Can you work these out from the model? Positions are in its coordinate system, mm. Face numbers are marked on the shaded views. A direction names the side the tool comes from. Round coordinates to 2 decimals unless told otherwise and drop trailing zeros. Order: outer loops, then holes, each group sorted by start corner. A loop starts at its lowest first (then second) coordinate and runs counter-clockwise, first axis right, second up. Notation, with made-up numbers: M -32,3 L 18,3 A16 cw 18,15 Z; hole C 57.25,60 d3. An arc over 180 degrees is marked long. Answer as a JSON object with one key per item and string values. Group by question number.
from build123d import *

# Parameters (mm, degrees)
SKETCH1_W           = 42.3
SKETCH1_H           = 42.3
BOSS_EXTRUDE1_DEPTH = 46.9
SKETCH2_W           = 39
SKETCH2_H           = 39
BOSS_EXTRUDE2_DEPTH = 4.85
SKETCH3_R           = 17.6
BOSS_EXTRUDE3_DEPTH = 15.88
SKETCH4_R           = 17.6
BOSS_EXTRUDE4_DEPTH = 6.5
SKETCH5_R           = 10.75
BOSS_EXTRUDE5_DEPTH = 2.15
SKETCH6_R           = 4
BOSS_EXTRUDE6_DEPTH = 17.5
CUT_EXTRUDE1_DEPTH  = 13.5
CHAMFER1_SIZE       = 3
CHAMFER2_SIZE       = 1
FILLET1_R           = 1


with BuildPart() as part:
    # Sketch1 → Boss-Extrude1 (new body)
    with BuildSketch(Plane.XY):
        Rectangle(SKETCH1_W, SKETCH1_H)
    extrude(amount=BOSS_EXTRUDE1_DEPTH)

    # Sketch2 → Boss-Extrude2 (add)
    with BuildSketch(Plane.XY.offset(46.9)):
        Rectangle(SKETCH2_W, SKETCH2_H)
    extrude(amount=BOSS_EXTRUDE2_DEPTH)

    # Sketch3 → Boss-Extrude3 (add)
    with BuildSketch(Plane.XY.offset(51.75)):
        Circle(SKETCH3_R)
    extrude(amount=BOSS_EXTRUDE3_DEPTH)

    # Sketch4 → Boss-Extrude4 (add)
    with BuildSketch(Plane.XY.offset(67.63)):
        Circle(SKETCH4_R)
    extrude(amount=BOSS_EXTRUDE4_DEPTH)

    # Sketch5 → Boss-Extrude5 (add)
    with BuildSketch(Plane.XY.offset(74.13)):
        with Locations(Location((0, 0, 0), (0, 0, 180))):
            Circle(SKETCH5_R)
    extrude(amount=BOSS_EXTRUDE5_DEPTH)

    # Sketch6 → Boss-Extrude6 (add)
    with BuildSketch(Plane.XY.offset(76.28)):
        Circle(SKETCH6_R)
    extrude(amount=BOSS_EXTRUDE6_DEPTH)

    # Sketch7 → Cut-Extrude1 (cut)
    with BuildSketch(Plane.XY.offset(93.78)):
        Polygon((-80.453133814, 3), (-2.645751311, 3), (2.645751311, 3), (80.453133814, 3), (80.453133814, 158.614765005), (-80.453133814, 158.614765005), align=None)
    extrude(amount=-CUT_EXTRUDE1_DEPTH, mode=Mode.SUBTRACT)

    # Chamfer1
    chamfer1_edges = [part.edges().sort_by_distance(p)[0] for p in [
        (19.5, -19.5, 49.325),
        (19.5, 19.5, 49.325),
        (-19.5, 19.5, 49.325),
        (-19.5, -19.5, 49.325),
        (-21.15, -21.15, 23.45),
        (21.15, -21.15, 23.45),
        (21.15, 21.15, 23.45),
        (-21.15, 21.15, 23.45),
    ]]
    chamfer(chamfer1_edges, length=CHAMFER1_SIZE)

    # Chamfer2
    chamfer2_edges = [part.edges().sort_by_distance(p)[0] for p in [
        (-19.5, 0, 51.75),
        (0, 19.5, 51.75),
        (19.5, 0, 51.75),
        (0, -19.5, 51.75),
        (18, 18, 51.75),
        (18, -18, 51.75),
        (-18, -18, 51.75),
        (-18, 18, 51.75),
    ]]
    chamfer(chamfer2_edges, length=CHAMFER2_SIZE)

    # Fillet1
    fillet1_edges = [part.edges().sort_by_distance(p)[0] for p in [
        (0, 3, 80.28),
    ]]
    fillet(fillet1_edges, radius=FILLET1_R - 0.0001)  # a hair under: the kernel refuses the full size


solid = part.part
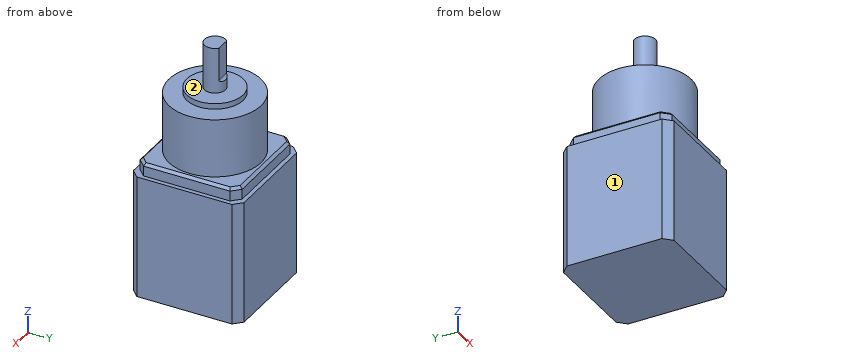
Item 1: Suppose I cut it at C-C, the plane y = -1. Write out the boundary of the cut face in (x, z), and give its area (3 significant figures).
Item 2: I'm going to push flat-ended pins straight in: pin 1 Ø8 at (x, y) = (-12, 10.5) entering from +Z; pin 2 Ø1.6 at (x, z) = (0, 86) entering from +Y; pin 3 Ø1 at (y, z) = (-13.5, 50) entering from -X. Where does each tip first touch, or does it pass through?
Item 3: Suppose I cut it at B-B, the plane z = 71. Write out the boundary of the cut face in (x, y).
Item 4: On a 3-axis mill with a long thin cutter (end or side, diameter ignored), from which of +Z, -Z, +X, -X, +Y, -Y can I reach the whole of each face in a straight line? I mean the marked faces 1 and 2. Say none if no direction works.
Item 5: Suppose I cut it at D-D, the plane y = 7.5. Write out the boundary of the cut face in (x, z).
Item 6: Suppose I cut it at A-A, the plane x = -9.5. Write out the boundary of the cut face in (y, z).
Item 7: I need wall thicknesses on line 1 (Z direction, x = -5, y = -7.5); line 2 (Z direction, x = 5, y = -17); line 3 (X direction, y = 13, z = 50). Which ranges of each line are inside material? Lowest first, please.
Computed:
{
 "1": {"outline": "M -21.15,0 L 21.15,0 L 21.15,46.9 L 19.5,46.9 L 19.5,50.75 L 18.5,51.75 L 17.57,51.75 L 17.57,74.13 L 10.7,74.13 L 10.7,76.28 L 3.87,76.28 L 3.87,93.78 L -3.87,93.78 L -3.87,76.28 L -10.7,76.28 L -10.7,74.13 L -17.57,74.13 L -17.57,51.75 L -18.5,51.75 L -19.5,50.75 L -19.5,46.9 L -21.15,46.9 Z", "area": "3,140 mm^2"},
 "2": {"pin 1": "stops at z = 74.13", "pin 2": "stops at y = 3", "pin 3": "stops at x = -19.5"},
 "3": {"outline": "C 0,0 d35.2"},
 "4": {"face 1": "+Z, -Z, -X, +Y, -Y", "face 2": "+Z"},
 "5": {"outline": "M -21.15,0 L 21.15,0 L 21.15,46.9 L 19.5,46.9 L 19.5,50.75 L 18.5,51.75 L 15.92,51.75 L 15.92,74.13 L 7.7,74.13 L 7.7,76.28 L -7.7,76.28 L -7.7,74.13 L -15.92,74.13 L -15.92,51.75 L -18.5,51.75 L -19.5,50.75 L -19.5,46.9 L -21.15,46.9 Z"},
 "6": {"outline": "M -21.15,0 L 21.15,0 L 21.15,46.9 L 19.5,46.9 L 19.5,50.75 L 18.5,51.75 L 14.82,51.75 L 14.82,74.13 L 5.03,74.13 L 5.03,76.28 L -5.03,76.28 L -5.03,74.13 L -14.82,74.13 L -14.82,51.75 L -18.5,51.75 L -19.5,50.75 L -19.5,46.9 L -21.15,46.9 Z"},
 "7": {"line 1": "z = 0 to 76.28", "line 2": "z = 0 to 51.75", "line 3": "x = -19.5 to 19.5"}
}
